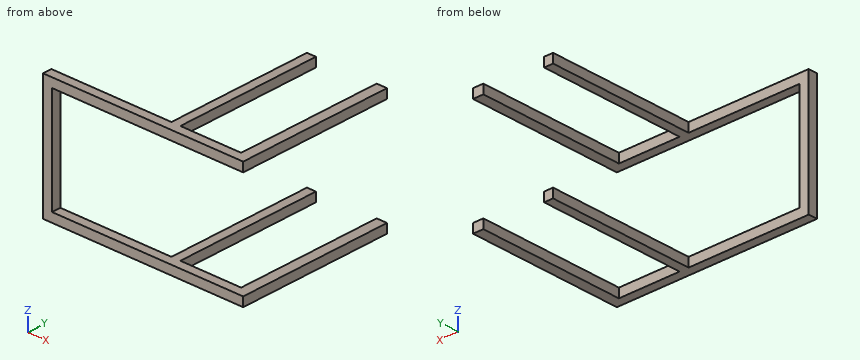
```python
from build123d import *

# Parameters (mm, degrees)
SALIENTE_EXTRUIR1_DEPTH = 58
CROQUIS3_W              = 58
CROQUIS3_H              = 58
CROQUIS3_W_2            = 66.947748122
SALIENTE_EXTRUIR2_DEPTH = 1000


with BuildPart() as part:
    # Croquis2 → Saliente-Extruir1 (new body)
    with BuildSketch(Plane(origin=(0, 0, 0), x_dir=(1, 0, 0), z_dir=(0, 1, 0))):
        Polygon((858.4, -333.5), (858.4, -391.5), (-435, -391.5), (-435, 391.5), (858.4, 391.5), (858.4, 333.5), (-377, 333.5), (-377, -333.5), align=None)
    extrude(amount=SALIENTE_EXTRUIR1_DEPTH)

    # Croquis3 → Saliente-Extruir2 (add)
    with BuildSketch(Plane(origin=(0, 0, 0), x_dir=(1, 0, 0), z_dir=(0, 1, 0))):
        with Locations((370, 362.5)):
            Rectangle(CROQUIS3_W, CROQUIS3_H)
        with Locations((824.926125939, 362.5)):
            Rectangle(CROQUIS3_W_2, CROQUIS3_H)
        with Locations((824.926125939, -362.5)):
            Rectangle(CROQUIS3_W_2, CROQUIS3_H)
        with Locations((370, -362.5)):
            Rectangle(CROQUIS3_W, CROQUIS3_H)
    extrude(amount=SALIENTE_EXTRUIR2_DEPTH)


solid = part.part
```
Could you check a few things on this model? Use its own coordinates, in mm. Coordinates: 2 decimals unless noted, no trailing zeros. Write each loop counter-clockwise with the first axis right and the second up, starting at its lowest first coordinate (ties: lowest second). Pieces come first, ordered by that corner, then holes. Notation, with made-up numbers: M -24.5,70 L -4.5,70 A31 cw -4.5,105 Z; hole C -37,10.25 d8. An arc over 180 degrees is marked long. Answer as CSV lines item,"result". Start each with the question number.
1) I want a section at B-B, the plane x = 626. Please give me the cut outline in (y, z).
2) Please list where these lines run through material, in increasing order: line 1 (X direction, y = 265, z = -360); line 2 (Z direction, x = 359, y = 240); line 3 (Y direction, x = -365.5, z = 341.5). Write a range as from..to.
3) I want a section at A-A, the plane y = 373. Please give me the cut outline in (x, z), and give its area (3 significant figures).
4) I want a section at C-C, the plane z = -127.5. Please give me the cut outline in (x, y).
Data:
1,outline,"M 0,-391.5 L 58,-391.5 L 58,-333.5 L 0,-333.5 Z; M 0,333.5 L 58,333.5 L 58,391.5 L 0,391.5 Z"
2,line 1,"x = 341..399, 791.45..858.4"
2,line 2,"z = -391.5..-333.5, 333.5..391.5"
2,line 3,"y = 0..58"
3,outline,"M 341,-391.5 L 399,-391.5 L 399,-333.5 L 341,-333.5 Z; M 341,333.5 L 399,333.5 L 399,391.5 L 341,391.5 Z; M 791.45,-391.5 L 858.4,-391.5 L 858.4,-333.5 L 791.45,-333.5 Z; M 791.45,333.5 L 858.4,333.5 L 858.4,391.5 L 791.45,391.5 Z"
3,area,"14,500 mm^2"
4,outline,"M -435,0 L -377,0 L -377,58 L -435,58 Z"
